Input: part model. Units: mm. Frame: model coordinates. Face numbers are marked on the shaded views. A direction names the side the tool comes from. Give positions to 0.01 mm unless a question says otherwise; leave off trailing zeros. Write each loop counter-clockwise with the first axis right and the second up, starting at its lowest first coordinate (ties: lowest second). Pieces come first, ordered by that corner, then holes. Notation, with made-up numbers: (30, 55) -> (65, 55) arc R11 cw to (65, 62) -> close; hole circle Ø11 at (-31.75, -20). An arc over 180 degrees is marked (long way). Return JSON: item names as keys, results as strings. Group by question number.
Item 1: Set-up query: the marked faces 5, 6, 7 and 8. Return all of +Z, -Z, +X, -X, +Y, -Y with unobstructed straight access to the full face (end or side cutting, diameter ignored); none if empty.
Item 2: Pin query (flat end, axial travel): P1, Ø5, axis at y = -16.5, z = 19, coming from the +X side; P2, Ø3, axis at y = 28.5, z = 8, coming from the +X side; P3, Ø3, axis at x = 21, z = 11, coming from the -Y side; P4, Ø12, axis at x = -13, z = 19, coming from the +Y side. Return the tip coordinate at first contact, or that it passes through.
Item 3: Section A-A, the plane z = 18.75. Return loops of the section in (x, y), then the cut area to 3 significant figures.
Item 4: Mould query, pull axis Y, two halves, no side actions, for the marked faces 1, 2, 3 and 4. Classes: released by +Y, released by -Y, zero draft, split by the parting line, or undercut.
Item 5: Line query: line 1 (Y direction, x = 0, z = 21); line 2 (X direction, y = 29, z = 6); line 3 (X direction, y = 6, z = 22). Output: solid intervals per line, ascending. Write a range as [from, to].
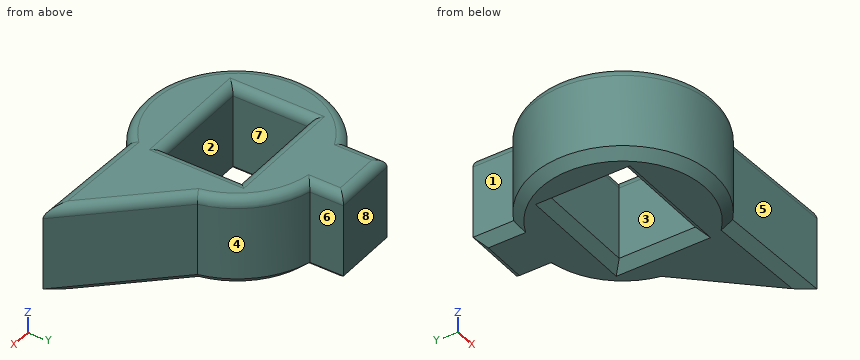
from build123d import *

# Parameters (mm, degrees)
F0_W     = 28.024344
F0_H     = 21.196416
F1_DEPTH = 25.4
F2_R     = 2.54
F3_SIZE  = 2.54


with BuildPart() as f1:
    # F0 (on Top) → F1 (new body)
    with BuildSketch(Plane.XY):
        with BuildLine():
            Line((-11.51223, 33.96108), (-11.51223, 22.641302))
            ThreePointArc((-11.51223, 22.641302), (-21.122827, -14.106246), (16.502721, -19.308552))
            Line((16.502721, -19.308552), (49.288545, -20.528002))
            Line((49.288545, -20.528002), (24.736057, 5.76953))
            ThreePointArc((24.736057, 5.76953), (18.164005, 17.754687), (6.331727, 24.598155))
            Line((6.331727, 24.598155), (6.331727, 33.96108))
            Line((6.331727, 33.96108), (-11.51223, 33.96108))
        make_face()
        Rectangle(F0_W, F0_H, mode=Mode.SUBTRACT)
    extrude(amount=F1_DEPTH)

    # F2
    f2_edges = [f1.edges().sort_by_distance(p)[0] for p in [
        (18.164005, 17.754687, 25.4),
        (6.331727, 29.279618, 25.4),
        (-2.590252, 33.96108, 25.4),
        (-11.51223, 28.301191, 25.4),
        (-21.122827, -14.106246, 25.4),
        (32.895633, -19.918277, 25.4),
        (37.012301, -7.379236, 25.4),
        (0, 10.598208, 25.4),
        (14.012172, 0, 25.4),
        (0, -10.598208, 25.4),
        (-14.012172, 0, 25.4),
    ]]
    fillet(f2_edges, radius=F2_R)

    # F3
    f3_edges = [f1.edges().sort_by_distance(p)[0] for p in [
        (18.164005, 17.754687, 0),
        (6.331727, 29.279618, 0),
        (-2.590252, 33.96108, 0),
        (-11.51223, 28.301191, 0),
        (-21.122827, -14.106246, 0),
        (32.895633, -19.918277, 0),
        (37.012301, -7.379236, 0),
        (0, 10.598208, 0),
        (14.012172, 0, 0),
        (0, -10.598208, 0),
        (-14.012172, 0, 0),
    ]]
    chamfer(f3_edges, length=F3_SIZE)


solid = f1.part
Answer below:
{
 "1": {"face 5": "+Z, -Z, -Y", "face 6": "+Z, -Z, +X, +Y", "face 7": "+Z, -Z", "face 8": "+Z, -Z, +X, -X, +Y"},
 "2": {"P1": "stops at x = 47.86", "P2": "stops at x = 6.33", "P3": "stops at y = -19.53", "P4": "stops at y = 33.96"},
 "3": {"outline": "(-11.51, 22.64) arc R25.4 ccw (long way) to (16.5, -19.31) -> (49.29, -20.53) -> (24.74, 5.77) arc R25.4 ccw to (6.33, 24.6) -> (6.33, 33.96) -> (-11.51, 33.96) -> close; hole (-14.01, -10.6) -> (14.01, -10.6) -> (14.01, 10.6) -> (-14.01, 10.6) -> close", "area": "1,950 mm2"},
 "4": {"face 1": "zero draft", "face 2": "undercut", "face 3": "undercut", "face 4": "released by +Y"},
 "5": {"line 1": "y = [-25.4, -10.6], [10.6, 33.96]", "line 2": "x = [-11.51, 6.33]", "line 3": "x = [-24.68, -14.01], [14.01, 24.68]"}
}
